Design review of the part built by this model. Coordinates are the model's own, in mm. Face numbers are marked on the shaded views. A direction names the side the tool comes from. Round coordinates to 2 decimals unless told otherwise and drop trailing zeros. Loops run counter-clockwise (first coordinate to the right, second up) from the corner with the lowest first, then second, coordinate; pieces in that order, holes last. Notation, with made-up numbers: M 3,27.5 L 54,27.5 A26 cw 54,41.5 Z; hole C -20.75,-9 d4. An arc over 180 degrees is marked long. Answer as CSV lines item,"result". Start each with the question number.
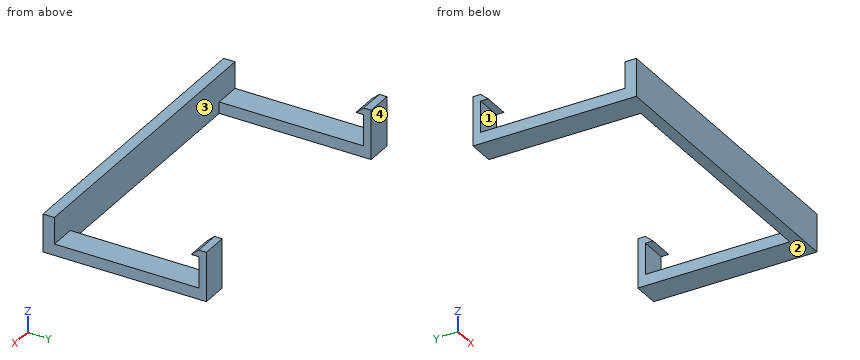
from build123d import *

# Parameters (mm, degrees)
BOSS_EXTRUDE1_DEPTH = 13
CUT_EXTRUDE1_DEPTH  = 100


with BuildPart() as part:
    # Sketch1 → Boss-Extrude1 (new body)
    with BuildSketch(Plane.XY):
        Polygon((0, 0), (40, 0), (40, 43), (33, 43), (33, 3), (0, 3), align=None)
    extrude(amount=BOSS_EXTRUDE1_DEPTH)

    # Sketch2 → Cut-Extrude1 (cut)
    with BuildSketch(Plane(origin=(40, 0, 0), x_dir=(0, 0, -1), z_dir=(1, 0, 0))):
        Polygon((-11.229441325, 39.002032062), (-13, 41), (-13, 0), (-10, 0), (-10, 3), (-3, 3), (-3, 41.002032062), (-11.229441325, 41.002032062), align=None)
    extrude(amount=-CUT_EXTRUDE1_DEPTH, mode=Mode.SUBTRACT)

    # Mirror2: part across plane


with BuildPart() as part_1:
    add(part.part)
    add(part.part.mirror(Plane(origin=(0, 0, 13), x_dir=(0, 0, 1), z_dir=(1, 0, 0))))


solid = part_1.part
Item 1: Tool access review of the marked faces 1 and 2: name each direction out of +Z, -Z, +X, -X, +Y, -Y from which nothing blocks a thin tool from reaching the whole face with its end or side.
Item 2: Consider section C-C, the plane z = 1.5. Write out the cut boundary in (x, y), then the cut area to 3 significant figures.
Item 3: Consider section D-D, the plane x = -5. Write out the cut boundary in (y, z).
Item 4: The part is to be moulded in two halves that separate along X. For the marked faces 3 and 4, say which applies: +X half, -X half, draft (parallel to the pull), parting line (faces both ways), or undercut.
Item 5: Insertion check: pin 1 Ø7.5 at (x, y) = (-36, 24) entering from +Z; pin 2 Ø4 at (x, z) = (-5.5, 3) entering from +Y; pin 3 Ø3.5 at (x, y) = (0.5, 1.5) entering from +Z; pin 4 Ø2 at (y, z) = (34, 5.5) entering from +X. Each pin has a flat end and moves straight along its axis. Give the tip position at first contact, or say it passes through.
Item 6: Consider section B-B, the plane y = 21. Write out the cut boundary in (x, z).
Item 7: Consider section A-A, the plane z = 6.75. Write out the cut boundary in (x, y).
Item 8: To check wall thickness, follow line 1 (X direction, y = 7, z = 1.25); line 2 (Y direction, x = -24.5, z = 2.5). State the ranges of each line that lie inside material, in increasing order.
Found:
1,face 1,"+X, -X"
1,face 2,"-Z, +X, -X, +Y, -Y"
2,outline,"M -40,0 L 40,0 L 40,43 L 33,43 L 33,3 L -33,3 L -33,43 L -40,43 Z"
2,area,"800 mm^2"
3,outline,"M 0,0 L 3,0 L 3,10 L 0,10 Z"
4,face 3,"undercut"
4,face 4,"draft"
5,pin 1,"stops at z = 3"
5,pin 2,"stops at y = 3"
5,pin 3,"stops at z = 10"
5,pin 4,"passes through"
6,outline,"M -40,0 L -33,0 L -33,3 L -40,3 Z; M 33,0 L 40,0 L 40,3 L 33,3 Z"
7,outline,"M -40,0 L 40,0 L 40,3 L -40,3 Z; M -40,41 L -33,41 L -33,43 L -40,43 Z; M 33,41 L 40,41 L 40,43 L 33,43 Z"
8,line 1,"x = -40 to -33, 33 to 40"
8,line 2,"y = 0 to 3"
